Geometry check sheet. Reference: the model listing, model coordinates, mm. Give positions to 0.01 mm unless a question says otherwise; leave off trailing zeros. Write each loop counter-clockwise with the first axis right and the second up, starting at its lowest first coordinate (ties: lowest second). Pieces come first, ordered by that corner, then holes. Notation, with made-up numbers: (83.25, 56) - (131.25, 56) arc R20 ccw to (131.25, 72) - close; hole circle Ø8 at (62, 68). An arc over 180 degrees is marked (long way). Use a Markdown table: item, result.
Autodesk Inventor part; units mm, degrees
ref_plane "YZ Plane" through (0, 0, 0) normal (1, 0, 0) x (0, 1, 0)
ref_plane "XZ Plane" through (0, 0, 0) normal (0, 1, 0) x (-1, 0, 0)
ref_plane "XY Plane" through (0, 0, 0) normal (0, 0, 1) x (1, 0, 0)
sketch "Sketch1" plane through (0, 0, 0) normal (0, 0, 1) x (1, 0, 0)
  line L0 (0, 0) -> (-25.4, 0)
  line L1 (-25.4, 0) -> (-25.4, 2.286)
  line L2 (-25.4, 2.286) -> (0, 2.286)
  line L3 (0, 2.286) -> (0, 0)
  line L4 (0, 0) -> (-2.286, 0)
  line L5 (-2.286, 0) -> (-2.286, 25.4)
  line L6 (-2.286, 25.4) -> (0, 25.4)
  line L7 (0, 25.4) -> (0, 0)
  dimension "d0" = 25.4
  dimension "d1" = 2.286
  dimension "d2" = 2.286
  dimension "d3" = 25.4
extrude "Extrusion1" add sketch "Sketch1" along normal blind 711.2
sketch "Sketch2" plane through (-25.4, 0, 0) normal (0, -1, 0) x (1, 0, 0)
  line L0 (0, 0) -> (25.4, 0)
  line L1 (25.4, 0) -> (25.4, 711.2)
  line L2 (0, 711.2) -> (25.4, 711.2)
  line L3 (0, 0) -> (0, 711.2)
  point P0 (12.7, 12.7)
  dimension "d6" = 12.7
  dimension "d7" = 12.7
hole "Hole1" at (-12.7, 0, 12.7) direction (0, 1, 0) diameter 3.9688 end through all
pattern_linear "Rectangular Pattern1" count 28 spacing 25.4 along (0, 0, 1) of "Hole1"
sketch "Sketch3" plane through (0, 0, 0) normal (1, 0, 0) x (0, 0, -1)
  line L0 (-711.2, 0) -> (-711.2, 25.4)
  line L1 (0, 0) -> (-711.2, 0)
  line L2 (0, 0) -> (0, 25.4)
  line L3 (0, 25.4) -> (-711.2, 25.4)
  point P0 (-12.7, 12.7)
  dimension "d18" = 12.7
  dimension "d19" = 12.7
hole "Hole2" at (0, 12.7, 12.7) direction (-1, 0, 0) diameter 3.9688 end through all
pattern_linear "Rectangular Pattern2" count 28 spacing 25.4 along (0, 0, 1) of "Hole2"
properties part number "bumper_angle"
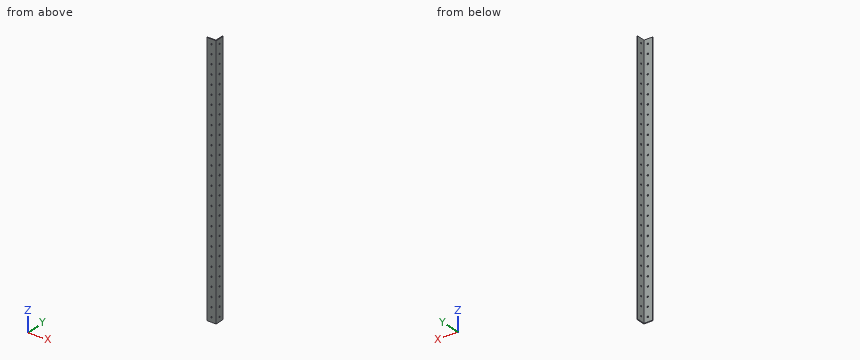
1) Section check B-B on y = 21.25. Record the boundary of the cut face in (x, z).
Working result:
| item | result |
|---|---|
| outline | (-2.29, 0) - (0, 0) - (0, 711.2) - (-2.29, 711.2) - close |
2) Material ranges on L1, parallel to X at y = 1.6, z = 38.1; L2, parallel to Y at x = -1.8, z = 266.7; L3, parallel to X at y = 5.5, z = 552, recorded low to high. Write a range as from..to.
Working result:
| item | result |
|---|---|
| L1 | x = -25.4..-14.68, -10.72..0 |
| L2 | y = 0..10.72, 14.68..25.4 |
| L3 | x = -2.29..0 |
3) Section check A-A on z = 102. Record the boundary of the cut face in (x, y).
Working result:
| item | result |
|---|---|
| outline | (-25.4, 0) - (0, 0) - (0, 25.4) - (-2.29, 25.4) - (-2.29, 2.29) - (-25.4, 2.29) - close |
4) Depth check by flat-ended pin: P1, Ø6.5, axis at x = -12.7, z = 292.1, coming from the -Y side; P2, Ø1, axis at y = 11, z = 212.5, coming from the -X side; P3, Ø6.5, axis at x = -12.7, z = 698.5, coming from the +Y side. Enter the tip coordinate at first touch or a pass-through.
Working result:
| item | result |
|---|---|
| P1 | stops at y = 0 |
| P2 | stops at x = -2.29 |
| P3 | stops at y = 2.29 |
5) Section check C-C on x = -21.25. Record the boundary of the cut face in (y, z), then the cut area to 3 significant figures.
Working result:
| item | result |
|---|---|
| outline | (0, 0) - (2.29, 0) - (2.29, 711.2) - (0, 711.2) - close |
| area | 1,630 mm² |
